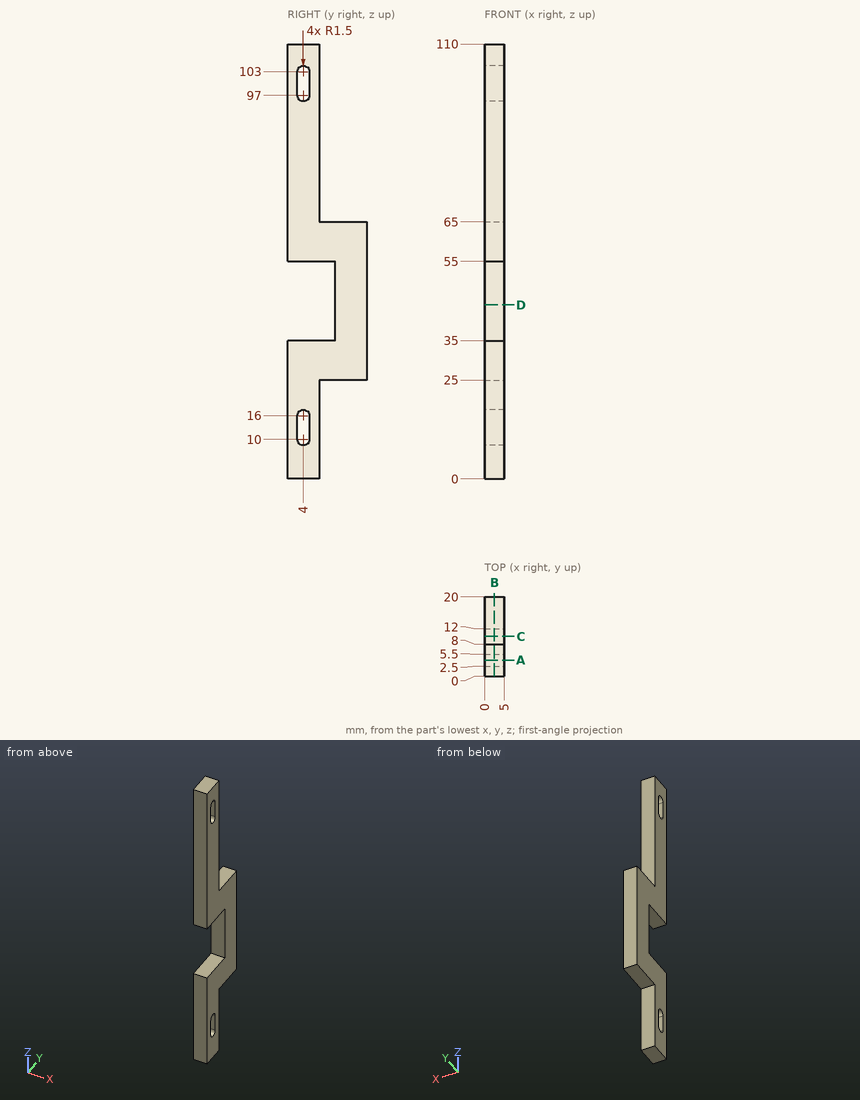
Geometry check sheet. Reference: drawing and pictorial views, mm from the part's lowest x, y, z. Give positions to 0.01 mm unless a question says otherwise; leave off trailing zeros. Order: outer loops, then holes, each group sorted by start corner. A loop starts at its lowest first (then second) coordinate and runs counter-clockwise, first axis right, second up. Notation, with made-up numbers: (-32, -28) -> (-13, -28) arc R26 ccw to (-13, -7) -> close; hole circle Ø6 at (64, 41). An arc over 180 degrees is marked (long way). Use CSV: the item, a comma, the result in double quotes. Start each with the question number.
1) Go/stop test with flat-tipped pins: P1, Ø1, axis at x = 1, y = 15, coming from the +Z side; P2, Ø2.5, axis at x = 3, z = 43, coming from the -Y side; P3, Ø2, axis at x = 1.5, z = 71, coming from the +Y side. Record where each tip stops, or that it passes through.
2) Sectioned sample at D-D, the plane z = 44. Record the boundary of the cut face in (x, y), plus the area to 3 significant figures.
3) Sectioned sample at B-B, the plane x = 2.45. Record the boundary of the cut face in (y, z).
4) Material ranges on line 1 (Z direction, x = 4.55, y = 10.25); line 2 (Z direction, x = 1.4, y = 3.5); line 3 (Z direction, x = 3.7, y = 1.5), recorded low to high. Write a range as from..to.
5) Sectioned sample at C-C, the plane y = 10. Record the boundary of the cut face in (x, z), plus the area to 3 significant figures.
6) Sectioned sample at A-A, the plane y = 4. Record the boundary of the cut face in (x, z).
Recorded:
1,P1,"z = 65"
1,P2,"y = 12"
1,P3,"y = 8"
2,outline,"(0, 12) -> (5, 12) -> (5, 20) -> (0, 20) -> close"
2,area,"40.0 mm2"
3,outline,"(0, 0) -> (8, 0) -> (8, 25) -> (20, 25) -> (20, 65) -> (8, 65) -> (8, 110) -> (0, 110) -> (0, 55) -> (12, 55) -> (12, 35) -> (0, 35) -> close; hole (2.5, 10) arc R1.5 ccw to (5.5, 10) -> (5.5, 16) arc R1.5 ccw to (2.5, 16) -> close; hole (2.5, 97) arc R1.5 ccw to (5.5, 97) -> (5.5, 103) arc R1.5 ccw to (2.5, 103) -> close"
4,line 1,"25..35, 55..65"
4,line 2,"0..8.59, 17.41..35, 55..95.59, 104.41..110"
4,line 3,"0..35, 55..110"
5,outline,"(0, 25) -> (5, 25) -> (5, 35) -> (0, 35) -> close; (0, 55) -> (5, 55) -> (5, 65) -> (0, 65) -> close"
5,area,"100 mm2"
6,outline,"(0, 0) -> (5, 0) -> (5, 8.5) -> (0, 8.5) -> close; (0, 17.5) -> (5, 17.5) -> (5, 35) -> (0, 35) -> close; (0, 55) -> (5, 55) -> (5, 95.5) -> (0, 95.5) -> close; (0, 104.5) -> (5, 104.5) -> (5, 110) -> (0, 110) -> close"
